Autodesk Inventor part; units mm, degrees
ref_plane "YZ Plane" through (0, 0, 0) normal (1, 0, 0) x (0, 1, 0)
ref_plane "XZ Plane" through (0, 0, 0) normal (0, 1, 0) x (-1, 0, 0)
ref_plane "XY Plane" through (0, 0, 0) normal (0, 0, 1) x (1, 0, 0)
sketch "Sketch1" plane through (0, 0, 0) normal (0, 0, 1) x (1, 0, 0)
  circle A0 centre (0, 0) radius 20
  dimension "d0" = 40
extrude "Extrusion1" add sketch "Sketch1" along normal blind 6.6
sketch "Sketch3" plane through (0, 0, 0) normal (0, 0, -1) x (-1, 0, 0)
  circle A0 centre (0, 0) radius 17
  line L0 (0, 17) -> (0, 0)
  line L1 (0, 0) -> (14.7224, -8.5)
  line L2 (0, 0) -> (-14.7224, -8.5)
  line L3 (0, 0) -> (17, 0) construction
  line L4 (1.5, 16.9337) -> (1.5, 0.866)
  line L5 (-1.5, 16.9337) -> (-1.5, 0.866)
  line L6 (-1.5, 0.866) -> (-15.415, -7.1678)
  line L7 (0, -1.7321) -> (-13.915, -9.7659)
  line L8 (1.5, 0.866) -> (15.415, -7.1678)
  line L9 (0, -1.7321) -> (13.915, -9.7659)
  dimension "d6" = 34
  dimension "d7" = 120
  dimension "d8" = 150
  dimension "d9" = 1.5
  dimension "d10" = 1.5
  dimension "d11" = 1.5
  dimension "d12" = 1.5
  dimension "d13" = 1.5
  dimension "d14" = 1.5
extrude "Extrusion3" cut sketch "Sketch3" against normal up to surface (6.6 mm away) contours A0 L8 L4 | L5 L6 A0 | A0 L7 L9
sketch "Sketch5" plane through (0, 0, 6.6) normal (0, 0, 1) x (1, 0, 0)
  circle A0 centre (0, 0) radius 4
  dimension "d20" = 8
extrude "Extrusion5" add sketch "Sketch5" against normal blind 6.6
sketch "Sketch6" plane through (0, 0, 0) normal (0, 0, -1) x (-1, 0, 0)
  circle A0 centre (0, 0) radius 2
  line L0 (0, -2) -> (0, -4)
  arc A1 (-2.4613, -3.1531) -> (2.4613, -3.1531) centre (0, 0) ccw
  line L1 (0.5, -1.9365) -> (0.5, -3.9686)
  line L2 (-0.5, -1.9365) -> (-0.5, -3.9686)
  line L3 (-1.3229, 1.5) -> (1.3229, 1.5)
  point P0 (0.0845, 1.5)
  dimension "d23" = 4
  dimension "d24" = 0.5
  dimension "d25" = 0.5
  dimension "d29" = 3.5
extrude "Extrusion6" cut sketch "Sketch6" against normal up to surface (6.6 mm away) contours A0 L3 | L1 A1 L0 A0 | L0 A1 L2 A0 picked at (-0.5622, -0.3103)
fillet "Arredondamento1" radius 1 2 edges at (-20, 0, 6.6) (-20, 0, 0)
properties part number "wheel4mmV1"
Check sheet for the modelled part. Datum: model origin and axes. Units: mm. A direction names the side the tool comes from. Coordinates: 2 decimals unless noted, no trailing zeros. Loops run counter-clockwise (first coordinate to the right, second up) from the corner with the lowest first, then second, coordinate; pieces in that order, holes last.
1) Gauge pin test, flat ends, axial feed: pin 1 (2 mm diameter, centred on y = -3, z = 4.5, fed in from -X); pin 2 (8 mm diameter, centred on x = 4.5, y = 15.5, fed in from +Z); pin 3 (1.5 mm diameter, centred on y = -11.5, z = 5.5, fed in from -X); pin 4 (0.6 mm diameter, centred on y = -2.5, z = 4, fed in from +X). Record the tip position at first contact, or that the pin passes through.
2) Release check for a two-part mould opening along Y. For faces 1 (the face through (1.5, 10, 3)), 2 (the face through (-4.336, 19.524, 3.268)), 3 (the face through (0, 3, 0)) record: released by +Y, released by -Y, zero draft, split by the parting line, or undercut.
3) Access from +Z, -Z, +X, -X, +Y, -Y to the whole of each face (thin tool, end or side, straight path). Record for faces 4 (the face through (0, 3, 6.6)), 5 (the face through (14.607, 8.697, 3.254)).
4) Sectioned sample at C-C (z = 2.75). Record the boundary of the cut face in (x, y) (1 decimal).
5) Sectioned sample at A-A (x = 0). Record the boundary of the cut face in (y, z).
6) Sectioned sample at D-D (y = 5). Count the separate pieces of the cut face and the enclosed holes in it, and give its area (3 significant figures).
7) Material ranges on probe 1 along X at (y, z) = (8, 6); probe 2 along Y at (x, z) = (-9, 0.75) (3 decimals); probe 3 along X at (y, z) = (7, 0.75), recorded low to high.
8) Sectioned sample at B-B (y = 0). Record the boundary of the cut face in (x, z), and give its area (3 significant figures).
Check sheet entries:
1. pin 1: stops at x = -19.9
1. pin 2: stops at z = 6.6
1. pin 3: stops at x = -16.87
1. pin 4: stops at x = 19.88
2. face 1: undercut
2. face 2: split by the parting line
2. face 3: zero draft
3. face 4: +Z, +X, -X, +Y, -Y
3. face 5: +Z, -Z
4. outline: circle Ø40 at (0, 0); hole (-15.4, -7.2) - (-4, -0.6) arc R4 cw to (-1.5, 3.7) - (-1.5, 16.9) arc R17 ccw to start; hole (-13.9, -9.8) arc R17 ccw to (13.9, -9.8) - (2.5, -3.2) arc R4 cw to (0.5, -4) - (0.5, -1.9) arc R2 ccw to (1.3, 1.5) - (-1.3, 1.5) arc R2 ccw to (-0.5, -1.9) - (-0.5, -4) arc R4 cw to (-2.5, -3.2) - close; hole (1.5, 3.7) arc R4 cw to (4, -0.6) - (15.4, -7.2) arc R17 ccw to (1.5, 16.9) - close
5. outline: (-20, 1) arc R1 ccw to (-19, 0) - (-17, 0) - (-17, 6.6) - (-19, 6.6) arc R1 ccw to (-20, 5.6) - close; (1.5, 0) - (19, 0) arc R1 ccw to (20, 1) - (20, 5.6) arc R1 ccw to (19, 6.6) - (1.5, 6.6) - close
6. separate pieces: 3
6. enclosed holes: 0
6. area: 60.1 mm2
7. probe 1: x = -18.24 to -15, -1.5 to 1.5, 15 to 18.24
7. probe 2: y = -17.825 to -14.422, -6.928 to -3.464, 14.422 to 17.825
7. probe 3: x = -18.7 to -15.49, -1.5 to 1.5, 15.49 to 18.7
8. outline: (-20, 1) arc R1 ccw to (-19, 0) - (-17, 0) - (-17, 6.6) - (-19, 6.6) arc R1 ccw to (-20, 5.6) - close; (-4, 0) - (-2, 0) - (-2, 6.6) - (-4, 6.6) - close; (2, 0) - (4, 0) - (4, 6.6) - (2, 6.6) - close; (17, 0) - (19, 0) arc R1 ccw to (20, 1) - (20, 5.6) arc R1 ccw to (19, 6.6) - (17, 6.6) - close
8. area: 65.1 mm2
